from build123d import *

# Parameters (mm, degrees)
F0_W      = 150
F0_H      = 65
F1_DEPTH  = 55
F2_W      = 5
F2_H      = 15
F3_DEPTH  = 150.001
F4_W      = 30
F4_H      = 40
F5_DEPTH  = 150.001
F6_SIZE   = 10
F7_R      = 20
F8_W      = 2.5
F8_H      = 43.3062759042
F9_DEPTH  = 150.001
F10_W     = 2.5
F10_H     = 43.4678007662
F11_DEPTH = 150.001
F12_R     = 15
F13_DEPTH = 25.001


with BuildPart() as f1:
    # F0 (on Front) → F1 (new body)
    with BuildSketch(Plane.XZ):
        Rectangle(F0_W, F0_H)
    extrude(amount=F1_DEPTH)

    # F2 (on face) → F3 (cut, through all)
    with BuildSketch(Plane.YZ.offset(75)):
        with Locations((-47.5, -25)):
            Rectangle(F2_W, F2_H)
    extrude(amount=-F3_DEPTH, mode=Mode.SUBTRACT)

    # F4 (on face) → F5 (cut, through all)
    with BuildSketch(Plane.YZ.offset(75)):
        with Locations((-27.5, 12.5)):
            Rectangle(F4_W, F4_H)
    extrude(amount=-F5_DEPTH, mode=Mode.SUBTRACT)

    # F6
    f6_edges = [f1.edges().sort_by_distance(p)[0] for p in [
        (75, -6.25, 32.5),
        (-75, -48.75, 32.5),
    ]]
    chamfer(f6_edges, length=F6_SIZE)

    # F7
    f7_edges = [f1.edges().sort_by_distance(p)[0] for p in [
        (75, -48.75, 32.5),
        (-75, -6.25, 32.5),
    ]]
    fillet(f7_edges, radius=F7_R)

    # F8 (on face) → F9 (cut, through all)
    with BuildSketch(Plane.YZ.offset(75)):
        with Locations((-53.75, 14.1531379521)):
            Rectangle(F8_W, F8_H)
    extrude(amount=-F9_DEPTH, mode=Mode.SUBTRACT)

    # F10 (on face) → F11 (cut, through all)
    with BuildSketch(Plane.YZ.offset(75)):
        with Locations((-1.25, 14.2339003831)):
            Rectangle(F10_W, F10_H)
    extrude(amount=-F11_DEPTH, mode=Mode.SUBTRACT)

    # F12 (on face) → F13 (cut, through all)
    with BuildSketch(Plane.XY.offset(-7.5)):
        with Locations((0, -27.5)):
            Circle(F12_R)
    extrude(amount=-F13_DEPTH, mode=Mode.SUBTRACT)


solid = f1.part
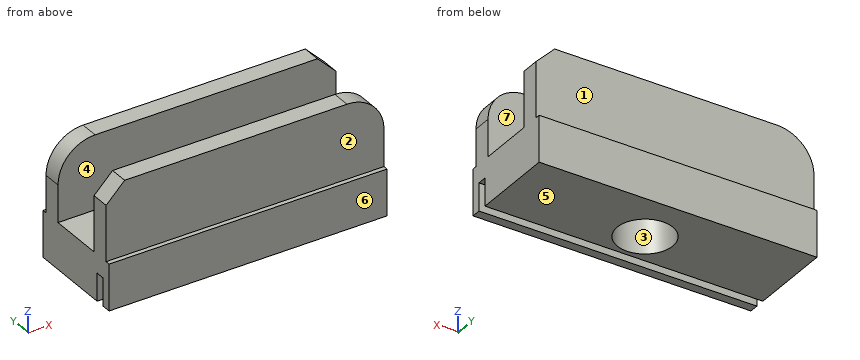
Check sheet for the modelled part. Datum: model origin and axes. Units: mm. Face numbers are marked on the shaded views. A direction names the side the tool comes from. Give positions to 0.01 mm unless a question says otherwise; leave off trailing zeros. Order: outer loops, then holes, each group sorted by start corner. A loop starts at its lowest first (then second) coordinate and runs counter-clockwise, first axis right, second up. Notation, with made-up numbers: M -3,14 L 51,14 A20 ccw 51,38 Z; hole C 85.25,-22.75 d10. An arc over 180 degrees is marked long. Answer as CSV lines item,"result". Start each with the question number.
Item 1: Cross-section at B-B on x = 8. Enter the section's corners in (y, z), plus the area to 3 significant figures.
Item 2: Thickness scan on line 1 (Y direction, x = 0, z = -24.25); line 2 (Y direction, x = 0, z = -14); line 3 (Y direction, x = 42, z = 7). Record the ranges inside material, lowest first. Write a range as [from, to].
Item 3: Mould release check, pull along Y, two halves, no side actions. Record for the marked faces 5, 6 and 7: +Y half, -Y half, draft (parallel to the pull), parting line (faces both ways), or undercut.
Item 4: Cross-section at A-A on z = 9. Enter the section's corners in (x, y).
Item 5: Cross-section at C-C on y = -27.5. Enter the section's corners in (x, z), plus the area to 3 significant figures.
Item 6: Cross-section at D-D on x = 32. Enter the section's corners in (y, z).
Item 7: Gauge pin test, flat ends, axial feed: P1, Ø3, axis at x = 25, z = 17.5, coming from the -Y side; P2, Ø6, axis at x = 54.5, y = -22, coming from the +Z side; P3, Ø20, axis at x = -9.5, z = 12.5, coming from the +Y side. Record the tip position at first contact, or that the pin passes through.
Item 8: Tool access check on the marked faces 1, 2, 3 and 4. Record the directions out of +Z, -Z, +X, -X, +Y, -Y that give a thin tool (end or side, any length) a straight path to the whole face; none if there is none.
Established:
1,outline,"M -55,-32.5 L -50,-32.5 L -50,-17.5 L -45,-17.5 L -45,-32.5 L -40.19,-32.5 L -40.19,-7.5 L -42.5,-7.5 L -42.5,32.5 L -52.5,32.5 L -52.5,-7.5 L -55,-7.5 Z; M -14.81,-32.5 L 0,-32.5 L 0,-7.5 L -2.5,-7.5 L -2.5,32.5 L -12.5,32.5 L -12.5,-7.5 L -14.81,-7.5 Z"
1,area,"1,470 mm^2"
2,line 1,"y = [-55, -50], [-45, -42.5], [-12.5, 0]"
2,line 2,"y = [-55, -42.5], [-12.5, 0]"
2,line 3,"y = [-52.5, -42.5], [-12.5, -2.5]"
3,face 5,"draft"
3,face 6,"-Y half"
3,face 7,"undercut"
4,outline,"M -75,-52.5 L 75,-52.5 L 75,-42.5 L -75,-42.5 Z; M -75,-12.5 L 75,-12.5 L 75,-2.5 L -75,-2.5 Z"
5,outline,"M -75,-32.5 L -15,-32.5 L -15,-7.5 L -75,-7.5 Z; M 15,-32.5 L 75,-32.5 L 75,-7.5 L 15,-7.5 Z"
5,area,"3,000 mm^2"
6,outline,"M -55,-32.5 L -50,-32.5 L -50,-17.5 L -45,-17.5 L -45,-32.5 L 0,-32.5 L 0,-7.5 L -2.5,-7.5 L -2.5,32.5 L -12.5,32.5 L -12.5,-7.5 L -42.5,-7.5 L -42.5,32.5 L -52.5,32.5 L -52.5,-7.5 L -55,-7.5 Z"
7,P1,"stops at y = -52.5"
7,P2,"stops at z = -7.5"
7,P3,"stops at y = -2.5"
8,face 1,"+Z, +X, -X, +Y"
8,face 2,"+Z, +X, -X, -Y"
8,face 3,"+Z, -Z"
8,face 4,"+Z, +X, -X"
